Verification items for the finished model (mm, model axes). A direction names the side the tool comes from. Give positions to 0.01 mm unless a question says otherwise; leave off trailing zeros. Write each loop counter-clockwise with the first axis right and the second up, starting at its lowest first coordinate (ties: lowest second). Pieces come first, ordered by that corner, then holes. Notation, with made-up numbers: (-24, 0) -> (18, 0) arc R22 ccw to (18, 23) -> close; hole circle Ø10 at (-2.5, 46.5). An arc over 180 degrees is marked (long way). Answer as CSV lines item,"result".
```python
from build123d import *

# Parameters (mm, degrees)
SKETCH1_W             = 50.8
SKETCH1_H             = 97.79
BOSS_EXTRUDE1_DEPTH   = 3
SKETCH2_W             = 10.16
SKETCH2_H             = 3
SKETCH2_W_2           = 3
SKETCH2_H_2           = 13.97
CUT_EXTRUDE1_DEPTH    = 4
F_8_CLEARANCE_HOLE2_D = 4.3053


with BuildPart() as part:
    # Sketch1 → Boss-Extrude1 (new body)
    with BuildSketch(Plane(origin=(0, 0, 0), x_dir=(1, 0, 0), z_dir=(0, 1, 0))):
        with Locations((25.4, 48.895)):
            Rectangle(SKETCH1_W, SKETCH1_H)
    extrude(amount=BOSS_EXTRUDE1_DEPTH)

    # Sketch2 → Cut-Extrude1 (cut, through all)
    with BuildSketch(Plane(origin=(0, 3, 0), x_dir=(1, 0, 0), z_dir=(0, 1, 0))):
        with Locations((15.24, 93.29)):
            Rectangle(SKETCH2_W, SKETCH2_H)
        with Locations((35.56, 93.29)):
            Rectangle(SKETCH2_W, SKETCH2_H)
        with Locations((49.3, 90.805)):
            Rectangle(SKETCH2_W_2, SKETCH2_H_2)
        with Locations((49.3, 62.865)):
            Rectangle(SKETCH2_W_2, SKETCH2_H_2)
        with Locations((49.3, 34.925)):
            Rectangle(SKETCH2_W_2, SKETCH2_H_2)
        with Locations((49.3, 6.985)):
            Rectangle(SKETCH2_W_2, SKETCH2_H_2)
        with Locations((35.56, 4.5)):
            Rectangle(SKETCH2_W, SKETCH2_H)
        with Locations((15.24, 4.5)):
            Rectangle(SKETCH2_W, SKETCH2_H)
        with Locations((1.5, 6.985)):
            Rectangle(SKETCH2_W_2, SKETCH2_H_2)
        with Locations((1.5, 34.925)):
            Rectangle(SKETCH2_W_2, SKETCH2_H_2)
        with Locations((1.5, 62.865)):
            Rectangle(SKETCH2_W_2, SKETCH2_H_2)
        with Locations((1.5, 90.805)):
            Rectangle(SKETCH2_W_2, SKETCH2_H_2)
    extrude(amount=-CUT_EXTRUDE1_DEPTH, mode=Mode.SUBTRACT)

    # #8 Clearance Hole2 (through all)
    with Locations(Plane(origin=(0, 3, 0), x_dir=(1, 0, 0), z_dir=(0, 1, 0))):
        with Locations((25.4, 48.895)):
            Hole(F_8_CLEARANCE_HOLE2_D / 2)


solid = part.part
```
1) Draft check along Z on faces 5 (the flat face through (3, 2, -35)), 6 (the flat face through (25, 1, 0)), 7 (the flat face through (1, 2, -83.82)). Enter one of: +Z half, -Z half, draft (parallel to the pull), parting line (faces both ways), or undercut.
Reported:
face 5,"undercut"
face 6,"+Z half"
face 7,"-Z half"
2) Section check C-C (z = -40.5). Record the boundary of the cut face in (x, y).
Reported:
outline,"(3, 0) -> (47.8, 0) -> (47.8, 3) -> (3, 3) -> close"
3) Scan lines: line 1 along Z through (x, y) = (39.5, 2.3); line 2 along Z through (x, y) = (2.5, 1.3); line 3 along X through (y, z) = (1.8, -93.5). Record each from-to range of solid material in increasing order.
Reported:
line 1,"-97.79 to -94.79, -91.79 to -6, -3 to 0"
line 2,"-83.82 to -69.85, -55.88 to -41.91, -27.94 to -13.97"
line 3,"3 to 10.16, 20.32 to 30.48, 40.64 to 47.8"
4) Tool access check on faces 1 (the flat face through (3, 2, -63)), 2 (the flat face through (47.8, 2, -35)), 3 (the flat face through (15, 2, -94.79)), 4 (the flat face through (1, 2, -13.97)). Record the directions out of +Z, -Z, +X, -X, +Y, -Y that give a thin tool (end or side, any length) a straight path to the whole face; none if there is none.
Reported:
face 1,"-X, +Y, -Y"
face 2,"+X, +Y, -Y"
face 3,"+Y, -Y"
face 4,"+Z, -X, +Y, -Y"
5) Section check B-B (x = 25.4). Record the boundary of the cut face in (y, z).
Reported:
outline,"(0, -97.79) -> (3, -97.79) -> (3, -51.05) -> (0, -51.05) -> close; (0, -46.74) -> (3, -46.74) -> (3, 0) -> (0, 0) -> close"
6) Section check A-A (x = 32). Record the boundary of the cut face in (y, z), and give its area (3 significant figures).
Reported:
outline,"(0, -97.79) -> (3, -97.79) -> (3, -94.79) -> (0, -94.79) -> close; (0, -91.79) -> (3, -91.79) -> (3, -6) -> (0, -6) -> close; (0, -3) -> (3, -3) -> (3, 0) -> (0, 0) -> close"
area,"275 mm²"
7) Section check D-D (y = 2.15). State how many separate pieces and enclosed holes the cut face has, and give its area (3 significant figures).
Reported:
separate pieces,"1"
enclosed holes,"5"
area,"4,500 mm²"
8) Depth check by flat-ended pin: pin 1 (1.5 mm diameter, centred on x = 2, y = 2, fed in from -Z); pin 2 (0.9 mm diameter, centred on x = 49.5, y = 1.5, fed in from +Z); pin 3 (6 mm diameter, centred on x = 9, z = -41, fed in from -Y); pin 4 (1.5 mm diameter, centred on y = 1.5, z = -5, fed in from -X). Enter the tip coordinate at first touch or a pass-through.
Reported:
pin 1,"z = -83.82"
pin 2,"z = -13.97"
pin 3,"y = 0"
pin 4,"x = 3"
